```python
from build123d import *

# Parameters (mm, degrees)
SKETCH1_W           = 25.5
SKETCH1_H           = 25.5
BOSS_EXTRUDE1_DEPTH = 25.5
SKETCH3_W           = 23.1
SKETCH3_H           = 23.1
BOSS_EXTRUDE2_DEPTH = 25
SKETCH5_W           = 23.1
SKETCH5_H           = 23.1
BOSS_EXTRUDE3_DEPTH = 25
SKETCH6_W           = 20
SKETCH6_H           = 20
CUT_EXTRUDE1_DEPTH  = 45.5
SKETCH7_W           = 20
SKETCH7_H           = 20
CUT_EXTRUDE2_DEPTH  = 45.5
FILLET1_R           = 1


with BuildPart() as part:
    # Sketch1 → Boss-Extrude1 (new body)
    with BuildSketch(Plane(origin=(0, 0, 0), x_dir=(1, 0, 0), z_dir=(0, 1, 0))):
        Rectangle(SKETCH1_W, SKETCH1_H)
    extrude(amount=BOSS_EXTRUDE1_DEPTH)

    # Sketch3 → Boss-Extrude2 (add)
    with BuildSketch(Plane(origin=(0, 25.5, 0), x_dir=(1, 0, 0), z_dir=(0, 1, 0))):
        Rectangle(SKETCH3_W, SKETCH3_H)
    extrude(amount=BOSS_EXTRUDE2_DEPTH)

    # Sketch5 → Boss-Extrude3 (add)
    with BuildSketch(Plane.XY.offset(12.75)):
        with Locations((0, 12.75)):
            Rectangle(SKETCH5_W, SKETCH5_H)
    extrude(amount=BOSS_EXTRUDE3_DEPTH)

    # Sketch6 → Cut-Extrude1 (cut)
    with BuildSketch(Plane.XY.offset(37.75)):
        with Locations((0, 12.75)):
            Rectangle(SKETCH6_W, SKETCH6_H)
    extrude(amount=-CUT_EXTRUDE1_DEPTH, mode=Mode.SUBTRACT)

    # Sketch7 → Cut-Extrude2 (cut)
    with BuildSketch(Plane(origin=(0, 50.5, 0), x_dir=(1, 0, 0), z_dir=(0, 1, 0))):
        Rectangle(SKETCH7_W, SKETCH7_H)
    extrude(amount=-CUT_EXTRUDE2_DEPTH, mode=Mode.SUBTRACT)

    # Fillet1
    fillet1_edges = [part.edges().sort_by_distance(p)[0] for p in [
        (11.55, 38, 11.55),
        (11.55, 38, -11.55),
        (-11.55, 38, -11.55),
        (-11.55, 38, 11.55),
        (11.55, 50.5, 0),
        (0, 50.5, -11.55),
        (-11.55, 50.5, 0),
        (0, 50.5, 11.55),
        (11.55, 1.2, 25.25),
        (11.55, 24.3, 25.25),
        (-11.55, 24.3, 25.25),
        (-11.55, 1.2, 25.25),
        (11.55, 12.75, 37.75),
        (0, 24.3, 37.75),
        (-11.55, 12.75, 37.75),
        (0, 1.2, 37.75),
    ]]
    fillet(fillet1_edges, radius=FILLET1_R)


solid = part.part
```
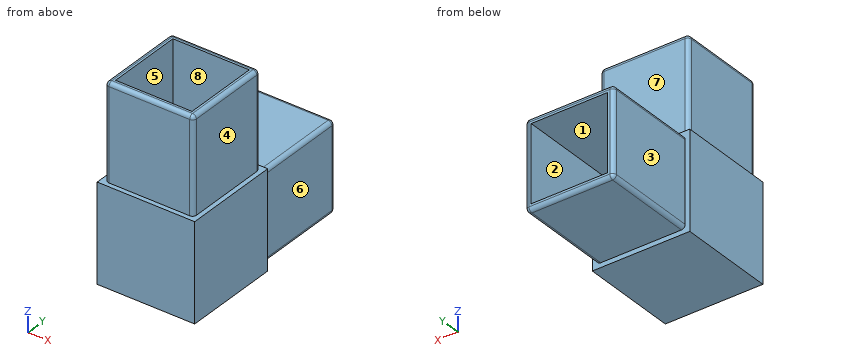
Geometry check sheet. Reference: the model listing, model coordinates, mm. Face numbers are marked on the shaded views. A direction names the side the tool comes from. Round coordinates to 2 decimals unless told otherwise and drop trailing zeros. Order: outer loops, then holes, each group sorted by start corner. A loop starts at its lowest first (then second) coordinate and runs counter-clockwise, first axis right, second up. Notation, with made-up numbers: (26.25, 36.5) - (82.25, 36.5) arc R31 cw to (82.25, 61.5) - close; hole circle Ø3 at (64, -30). An arc over 180 degrees is marked (long way). Use a Markdown table: item, result. Add a question column.
(1) Depth check by flat-ended pin: pin 1 (17 mm diameter, centred on y = 36, z = -2, fed in from -X); pin 2 (5 mm diameter, centred on x = 3.5, y = 34.5, fed in from +Z); pin 3 (6.5 mm diameter, centred on x = -2, z = 24, fed in from -Y). Enter the tip coordinate at first touch or a pass-through.
(2) Material ranges on line 1 along Z through (x, y) = (8.25, 32.5); line 2 along X through (y, z) = (7.5, -3.5); line 3 along Y through (x, z) = (-8.75, 33.5), recorded low to high. Write a range as [from, to].
(3) Sectioned sample at B-B, the plane z = 30. Enter the section's corners in (x, y).
(4) Release check for a two-part mould opening along X. For the marked faces 1, 2, 3 and 4 record: pulls with the +X half, pulls with the -X half, needs draft (parallel to the pull), parting line crosses it, or undercut.
(5) Tool access check on the marked faces 5, 6, 7 and 8. Record the directions out of +Z, -Z, +X, -X, +Y, -Y that give a thin tool (end or side, any length) a straight path to the whole face; none if there is none.
(6) Sectioned sample at A-A, the plane y = 31. Enter the section's corners in (x, z), and give its area (3 significant figures).
(7) Sectioned sample at C-C, the plane x = 3.25. Enter the section's corners in (y, z).
(8) Sectioned sample at D-D, the plane y = 4. Enter the section's corners in (x, z), and give its area (3 significant figures).
Answers below:
| question | item | result |
|---|---|---|
| 1 | pin 1 | x = -11.55 |
| 1 | pin 2 | z = 11.55 |
| 1 | pin 3 | y = 1.2 |
| 2 | line 1 | [-11.55, -10], [10, 11.55] |
| 2 | line 2 | [-12.75, -10], [10, 12.75] |
| 2 | line 3 | [1.2, 2.75], [22.75, 24.3] |
| 3 | outline | (-11.55, 2.2) arc R1 ccw to (-10.55, 1.2) - (10.55, 1.2) arc R1 ccw to (11.55, 2.2) - (11.55, 23.3) arc R1 ccw to (10.55, 24.3) - (-10.55, 24.3) arc R1 ccw to (-11.55, 23.3) - close; hole (-10, 2.75) - (10, 2.75) - (10, 22.75) - (-10, 22.75) - close |
| 4 | face 1 | undercut |
| 4 | face 2 | undercut |
| 4 | face 3 | pulls with the -X half |
| 4 | face 4 | pulls with the +X half |
| 5 | face 5 | none |
| 5 | face 6 | +Z, -Z, +X, +Y |
| 5 | face 7 | +Z, +X, -X, +Y |
| 5 | face 8 | +Z |
| 6 | outline | (-11.55, -10.55) arc R1 ccw to (-10.55, -11.55) - (10.55, -11.55) arc R1 ccw to (11.55, -10.55) - (11.55, 10.55) arc R1 ccw to (10.55, 11.55) - (-10.55, 11.55) arc R1 ccw to (-11.55, 10.55) - close; hole (-10, -10) - (10, -10) - (10, 10) - (-10, 10) - close |
| 6 | area | 133 mm² |
| 7 | outline | (0, -12.75) - (25.5, -12.75) - (25.5, -11.55) - (49.5, -11.55) arc R1 ccw to (50.5, -10.55) - (50.5, -10) - (5, -10) - (5, -7.75) - (2.75, -7.75) - (2.75, 37.75) - (2.2, 37.75) arc R1 ccw to (1.2, 36.75) - (1.2, 12.75) - (0, 12.75) - close; (22.75, 10) - (50.5, 10) - (50.5, 10.55) arc R1 ccw to (49.5, 11.55) - (25.5, 11.55) - (25.5, 12.75) - (24.3, 12.75) - (24.3, 36.75) arc R1 ccw to (23.3, 37.75) - (22.75, 37.75) - close |
| 8 | outline | (-12.75, -12.75) - (12.75, -12.75) - (12.75, 12.75) - (11.55, 12.75) - (11.55, 36.75) arc R1 ccw to (10.55, 37.75) - (10, 37.75) - (10, -7.75) - (-10, -7.75) - (-10, 37.75) - (-10.55, 37.75) arc R1 ccw to (-11.55, 36.75) - (-11.55, 12.75) - (-12.75, 12.75) - close |
| 8 | area | 317 mm² |
